Here's the drawing with two shaded views (mm, measured from the low corner). I have some questions. A direction names the side the tool comes from. Give positions to 0.01 mm unless a question says otherwise; leave off trailing zeros. Loops run counter-clockwise (first coordinate to the right, second up) from the corner with the lowest first, then second, coordinate; pieces in that order, holes last. Notation, with made-up numbers: M 0.5,28 L 19.5,28 A24 cw 19.5,55 Z; hole C 84.25,50.25 d3. An arc over 180 degrees is marked long. Answer in a Markdown table with one row per item. Add a question column.
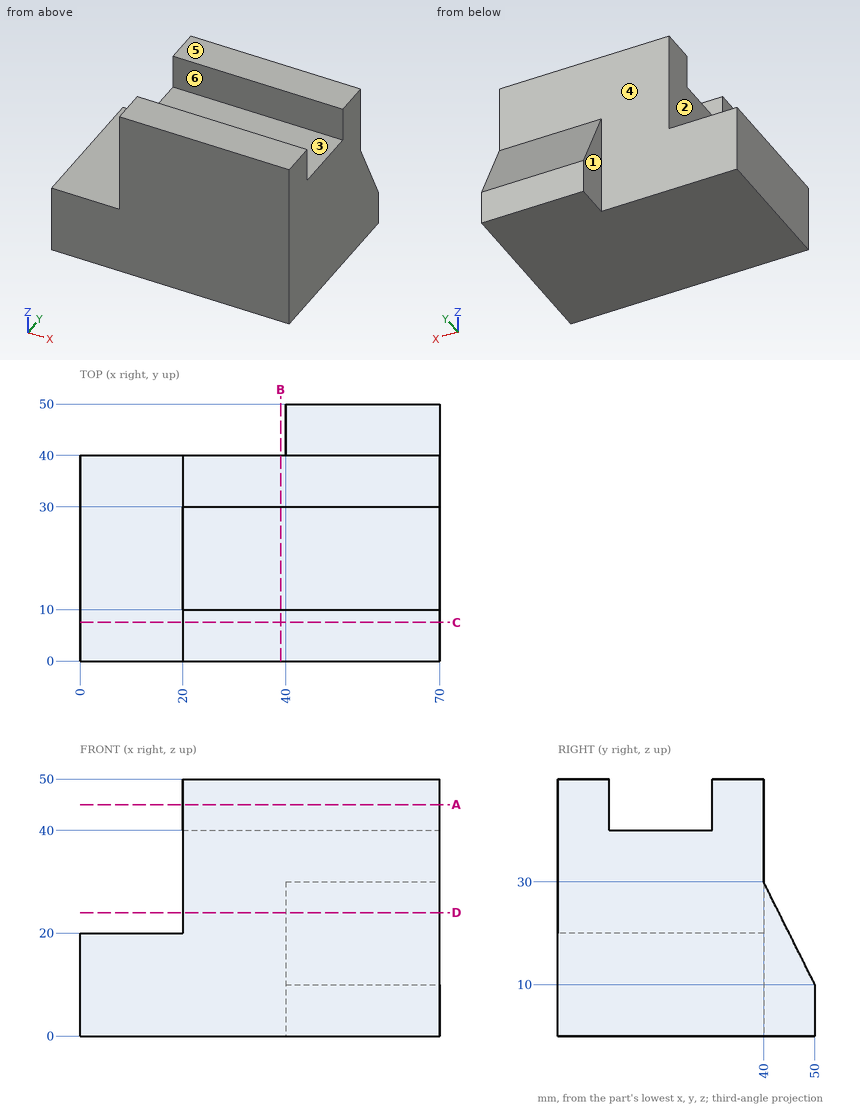
Item 1: Suppose I cut it at C-C (y = 7.5). List the corners of the cut face in (x, z) for me, then the cut area to 3 significant figures.
Item 2: For P1, Ø1, axis at x = 35, z = 29, coming from the +Y side; P2, Ø22, axis at x = 7, y = 20, coming from the +Z side, each with a flat end and sliding along its axis, tell me the tip position at first contact or that it passes through.
Item 3: For the marked faces 1, 2 and 3, which set-ups out of +Z, -Z, +X, -X, +Y, -Y let a thin tool reach every point of the face, with its end or its side?
Item 4: I need wall thicknesses on L1, parallel to Y at x = 54, z = 43; L2, parallel to Z at x = 33.5, y = 17. Which ranges of each line are inside material? Lowest first, please.
Item 5: Suppose I cut it at A-A (z = 45). List the corners of the cut face in (x, y) for me.
Item 6: Suppose I cut it at B-B (x = 39). List the corners of the cut face in (y, z) for me.
Item 7: Suppose I cut it at D-D (z = 24). List the corners of the cut face in (x, y) for me.
Item 8: If we mould it in two halves opening along Y, with no side actions, what happens to the marked faces 4, 5 and 6? For each: +Y half, -Y half, draft (parallel to the pull), parting line (faces both ways), or undercut.
Values found:
| question | item | result |
|---|---|---|
| 1 | outline | M 0,0 L 70,0 L 70,50 L 20,50 L 20,20 L 0,20 Z |
| 1 | area | 2,900 mm² |
| 2 | P1 | y = 40 |
| 2 | P2 | z = 20 |
| 3 | face 1 | +Z, -Z, -X, +Y |
| 3 | face 2 | +Z, -X, +Y, -Y |
| 3 | face 3 | +Z, +X, -X |
| 4 | L1 | 0 to 10, 30 to 40 |
| 4 | L2 | 0 to 40 |
| 5 | outline | M 20,0 L 70,0 L 70,10 L 20,10 Z; M 20,30 L 70,30 L 70,40 L 20,40 Z |
| 6 | outline | M 0,0 L 40,0 L 40,50 L 30,50 L 30,40 L 10,40 L 10,50 L 0,50 Z |
| 7 | outline | M 20,0 L 70,0 L 70,43 L 40,43 L 40,40 L 20,40 Z |
| 8 | face 4 | +Y half |
| 8 | face 5 | draft |
| 8 | face 6 | undercut |
